```python
from build123d import *

# Parameters (mm, degrees)
SKETCH1_R           = 9.525
SKETCH1_R_2         = 8.382
BOSS_EXTRUDE1_DEPTH = 260.35
SKETCH2_R           = 3
CUT_EXTRUDE1_DEPTH  = 20.05


with BuildPart() as part:
    # Sketch1 → Boss-Extrude1 (new body)
    with BuildSketch(Plane.XY):
        Circle(SKETCH1_R)
        Circle(SKETCH1_R_2, mode=Mode.SUBTRACT)
    extrude(amount=BOSS_EXTRUDE1_DEPTH)

    # Sketch2 → Cut-Extrude1 (cut, through all)
    with BuildSketch(Plane(origin=(9.525, 0, 0), x_dir=(0, 0, -1), z_dir=(1, 0, 0))):
        with Locations((-254, 0)):
            Circle(SKETCH2_R)
        with Locations((-6.35, 0)):
            Circle(SKETCH2_R)
    extrude(amount=-CUT_EXTRUDE1_DEPTH, mode=Mode.SUBTRACT)


solid = part.part
```
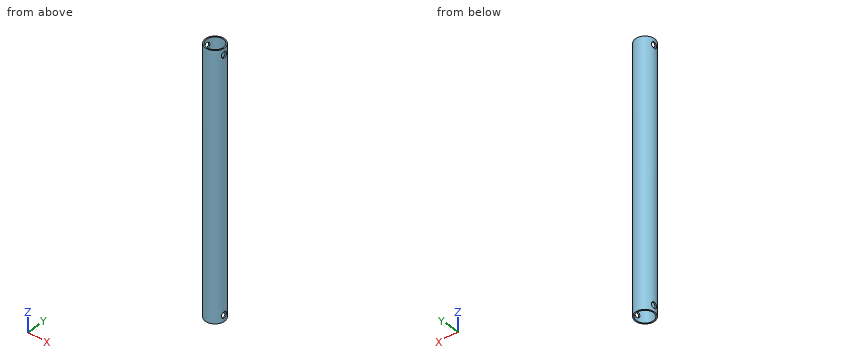
Geometry: final body of the model. Coordinates: model frame, mm. Coordinates: 2 decimals unless noted, no trailing zeros. Order: outer loops, then holes, each group sorted by start corner. A loop starts at its lowest first (then second) coordinate and runs counter-clockwise, first axis right, second up. Notation, with made-up numbers: M -37.5,24.25 L -24.5,24.25 A21 cw -24.5,47.25 Z; hole C 66.25,30 d7. An arc over 180 degrees is marked long. Answer as CSV lines item,"result".
Q1. First-contact query: P1, Ø8, axis at y = 6, z = 168.5, coming from the -X side; P2, Ø10, axis at x = -6.5, z = 230.5, coming from the -Y side; P3, Ø5, axis at x = -3.5, z = 204, coming from the +Y side. Flat tips, straight axial feed; report the tip coordinate or a pass-through.
Answers:
P1,"stops at x = -9.31"
P2,"stops at y = -9.41"
P3,"stops at y = 9.47"
Q2. Section B-B on z = 254. Return the cut outline in (x, y) (3 decimals), and give its area (3 significant figures).
Answers:
outline,"M -9.04,-3 A9.525 ccw 9.04,-3 L 7.827,-3 A8.382 cw -7.827,-3 Z; M -9.04,3 L -7.827,3 A8.382 cw 7.827,3 L 9.04,3 A9.525 ccw Z"
area,"50.3 mm^2"
Q3. Section D-D on z = 131.5. Return the cut outline in (x, y) (3 decimals), and give its area (3 significant figures).
Answers:
outline,"C 0,0 d19.05; hole C 0,0 d16.764"
area,"64.3 mm^2"
Q4. Section C-C on x = 3. Return the cut outline in (y, z), and give its area (3 significant figures).
Answers:
outline,"M -9.04,0 L -7.83,0 L -7.83,260.35 L -9.04,260.35 Z; M 7.83,0 L 9.04,0 L 9.04,260.35 L 7.83,260.35 Z"
area,"632 mm^2"
Q5. Section A-A on y = 0. Return the cut outline in (x, z) (3 decimals).
Answers:
outline,"M -9.525,0 L -8.382,0 L -8.382,3.35 L -9.525,3.35 Z; M -9.525,9.35 L -8.382,9.35 L -8.382,251 L -9.525,251 Z; M -9.525,257 L -8.382,257 L -8.382,260.35 L -9.525,260.35 Z; M 8.382,0 L 9.525,0 L 9.525,3.35 L 8.382,3.35 Z; M 8.382,9.35 L 9.525,9.35 L 9.525,251 L 8.382,251 Z; M 8.382,257 L 9.525,257 L 9.525,260.35 L 8.382,260.35 Z"
Q6. Line query: probe 1 along Z at (x, y) = (8.95, 0); probe 2 along X at (y, z) = (7.75, 128); probe 3 along Y at (x, z) = (-3.75, 113). Output: solid intervals per line, ascending. Write a range as [from, to].
Answers:
probe 1,"z = [0, 3.35], [9.35, 251], [257, 260.35]"
probe 2,"x = [-5.54, -3.19], [3.19, 5.54]"
probe 3,"y = [-8.76, -7.5], [7.5, 8.76]"
